```python
from build123d import *

# Parameters (mm, degrees)
RESSALTO_EXTRUS_O1_DEPTH = 12
ESBO_O2_W                = 27.357600802
ESBO_O2_H                = 15.919060402
CORTE_EXTRUS_O1_DEPTH    = 7.5
FILETE1_R                = 3
ESBO_O3_R                = 2.25
CORTE_EXTRUS_O2_DEPTH    = 2.5
FILETE2_R                = 3
ESBO_O4_R                = 1
CORTE_EXTRUS_O3_DEPTH    = 33.811931028


with BuildPart() as part:
    # Esboço1 → Ressalto-extrusão1 (new body)
    with BuildSketch(Plane.XY):
        with BuildLine():
            Line((21.183373259, 3.5), (0, 3.5))
            ThreePointArc((0, 3.5), (-3.5, 0), (0, -3.5))
            Line((0, -3.5), (23.285443563, -3.5))
            Line((23.285443563, -3.5), (28.893826204, -5.90573293))
            Line((28.893826204, -5.90573293), (30.943148627, 0.251790361))
            Line((30.943148627, 0.251790361), (21.183373259, 3.5))
        make_face()
    extrude(amount=RESSALTO_EXTRUS_O1_DEPTH)

    # Esboço2 → Corte-extrusão1 (cut)
    with BuildSketch(Plane(origin=(0, 0, 0), x_dir=(-1, 0, 0), z_dir=(0, 0, -1))):
        with Locations((-7.389764087, -0.137286393)):
            Rectangle(ESBO_O2_W, ESBO_O2_H)
    extrude(amount=-CORTE_EXTRUS_O1_DEPTH, mode=Mode.SUBTRACT)

    # Filete1
    filete1_edges = [part.edges().sort_by_distance(p)[0] for p in [
        (30.943148627, 0.251790361, 6),
        (28.893826204, -5.90573293, 6),
    ]]
    fillet(filete1_edges, radius=FILETE1_R)

    # Esboço3 → Corte-extrusão2 (cut)
    with BuildSketch(Plane(origin=(0, 0, 7.5), x_dir=(-1, 0, 0), z_dir=(0, 0, -1))):
        Circle(ESBO_O3_R)
    extrude(amount=-CORTE_EXTRUS_O2_DEPTH, mode=Mode.SUBTRACT)

    # Filete2
    filete2_edges = [part.edges().sort_by_distance(p)[0] for p in [
        (21.068564488, 0, 7.5),
        (21.068564488, 0, 0),
    ]]
    fillet(filete2_edges, radius=FILETE2_R)

    # Esboço4 → Corte-extrusão3 (cut, through all)
    with BuildSketch(Plane.XY.offset(12)):
        Circle(ESBO_O4_R)
    extrude(amount=-CORTE_EXTRUS_O3_DEPTH, mode=Mode.SUBTRACT)


solid = part.part
```
Geometry: final body of the model. Coordinates: model frame, mm. A direction names the side the tool comes from. Give positions to 0.01 mm unless a question says otherwise; leave off trailing zeros. Write each loop counter-clockwise with the first axis right and the second up, starting at its lowest first coordinate (ties: lowest second). Pieces come first, ordered by that corner, then holes.
1. Section query C-C, the plane z = 6.75. Return loops of the section in (x, y).
2. Section query B-B, the plane y = 0. Return loops of the section in (x, z), then the cut area to 3 significant figures.
3. Line query: probe 1 along Z at (x, y) = (16, 1.5); probe 2 along Y at (x, z) = (-0.5, 8.5); probe 3 along Y at (x, z) = (5, 11.25). Output: solid intervals per line, ascending.
4. Section query D-D, the plane y = 1.75. Return loops of the section in (x, z).
5. Reachability of faces 1 (the flat face through (1, -1, 10)), 2 (the flat face through (14, -3.5, 9)), 3 (the flat face through (21.069, 0, 4)) from +Z, -Z, +X, -X, +Y, -Y: full face, straight path, thin tool, end or side. Return the list, or none.
6. Section query A-A, the plane z = 8.25. Return loops of the section in (x, y).
7. Pin query (flat end, axial travel): P1, Ø5, axis at x = 21, z = 4.5, coming from the +Y side; P2, Ø2, axis at x = 1, y = -1, coming from the -Z side; P3, Ø2.5, axis at x = 0, y = 0, coming from the -Z side; P4, Ø2, axis at y = 0.5, z = 10.5, coming from the +X side. Return the tip coordinate at first contact, or that it passes through.
Computed:
1. outline: (20.05, -3.5) - (23.29, -3.5) - (25.9, -4.62) arc R3 ccw to (29.92, -2.81) - (30, -2.59) arc R3 ccw to (28.1, 1.2) - (21.18, 3.5) - (20.05, 3.5) - close
2. outline: (-3.5, 7.5) - (-2.25, 7.5) - (-2.25, 10) - (-1, 10) - (-1, 12) - (-3.5, 12) - close; (1, 10) - (2.25, 10) - (2.25, 7.5) - (18.07, 7.5) arc R3 cw to (21.07, 4.5) - (21.07, 3) arc R3 ccw to (24.07, 0) - (29.66, 0) - (29.66, 12) - (1, 12) - close
2. area: 198 mm2
3. probe 1: z = 7.5 to 12
3. probe 2: y = -3.46 to -2.19, 2.19 to 3.46
3. probe 3: y = -3.5 to 3.5
4. outline: (-3.03, 7.5) - (-1.41, 7.5) - (-1.41, 10) - (1.41, 10) - (1.41, 7.5) - (18.07, 7.5) arc R3 cw to (21.07, 4.5) - (21.07, 3) arc R3 ccw to (24.07, 0) - (26.44, 0) - (26.44, 12) - (-3.03, 12) - close
5. face 1: -Z
5. face 2: +Z, -Z, -X, -Y
5. face 3: -Z, -X, +Y, -Y
6. outline: (0, -3.5) - (23.29, -3.5) - (25.9, -4.62) arc R3 ccw to (29.92, -2.81) - (30, -2.59) arc R3 ccw to (28.1, 1.2) - (21.18, 3.5) - (0, 3.5) arc R3.5 ccw to start; hole circle Ø4.5 at (0, 0)
7. P1: stops at y = 3.5
7. P2: stops at z = 7.5
7. P3: stops at z = 10
7. P4: stops at x = 29.92
